Model file for the job. Use its own axes, mm. A direction names the side the tool comes from. Round coordinates to 2 decimals unless told otherwise and drop trailing zeros. Write each loop counter-clockwise with the first axis right and the second up, starting at its lowest first coordinate (ties: lowest second). Pieces come first, ordered by that corner, then holes. Notation, with made-up numbers: (77.5, 80) - (93.5, 80) arc R29 cw to (93.5, 108) - close; hole circle Ø9 at (-37.75, 24.5). An arc over 180 degrees is marked (long way). One line per item, written item: value.
from build123d import *

# Parameters (mm, degrees)
F1_DEPTH = 7.5
F2_W     = 18
F2_H     = 4
F2_W_2   = 8
F3_DEPTH = 7.5
F4_DEPTH = 5
F5_DEPTH = 25
F6_DEPTH = 3.5
F7_DEPTH = 25
F8_R     = 7
F9_R     = 1.99999


# Not quite as in the source:
# - a fillet or chamfer is up to 0.001 mm smaller than in the source, because OpenCascade refuses the exact size


with BuildPart() as f1:
    # F0 (on Top) → F1 (new body, symmetric)
    with BuildSketch(Plane.XY):
        Polygon((29.4704200836, 10.5355388032), (29.4704200836, 14.5355388032), (-5.5295799164, 14.5355388032), (-5.5295799164, -27.9644611968), (29.4704200836, -27.9644611968), (29.4704200836, -23.9644611968), (27.4704200836, -23.9644611968), (-1.5295799164, -23.9644611968), (-1.5295799164, 10.5355388032), (27.4704200836, 10.5355388032), align=None)
    extrude(amount=F1_DEPTH, both=True)

    # F2 (on Top) → F3 (join, symmetric)
    with BuildSketch(Plane.XY):
        Polygon((-30.5295799164, 18.5355388032), (-30.5295799164, 64.5355388032), (-18.5295799164, 64.5355388032), (-18.5295799164, 68.5355388032), (-34.5295799164, 68.5355388032), (-34.5295799164, 14.5355388032), (-23.5295799164, 14.5355388032), (-23.5295799164, 18.5355388032), align=None)
        Polygon((-10.5295799164, 68.5355388032), (-10.5295799164, 64.5355388032), (15.4704200836, 64.5355388032), (15.4704200836, 18.5355388032), (-5.5295799164, 18.5355388032), (-5.5295799164, 14.5355388032), (19.4704200836, 14.5355388032), (19.4704200836, 68.5355388032), align=None)
        with Locations((-14.5295799164, 16.5355388032)):
            Rectangle(F2_W, F2_H)
        with Locations((-14.5295799164, 66.5355388032)):
            Rectangle(F2_W_2, F2_H)
    extrude(amount=F3_DEPTH, both=True)

    # F2 (on Top) → F4 (cut, symmetric)
    with BuildSketch(Plane.XY):
        with Locations((-14.5295799164, 16.5355388032)):
            Rectangle(F2_W, F2_H)
    extrude(amount=F4_DEPTH, both=True, mode=Mode.SUBTRACT)

    # F2 (on Top) → F5 (cut)
    with BuildSketch(Plane.XY):
        with Locations((-14.5295799164, 16.5355388032)):
            Rectangle(F2_W, F2_H)
    extrude(amount=-F5_DEPTH, mode=Mode.SUBTRACT)

    # F2 (on Top) → F6 (cut, symmetric)
    with BuildSketch(Plane.XY):
        with Locations((-14.5295799164, 66.5355388032)):
            Rectangle(F2_W_2, F2_H)
    extrude(amount=F6_DEPTH, both=True, mode=Mode.SUBTRACT)

    # F2 (on Top) → F7 (cut)
    with BuildSketch(Plane.XY):
        with Locations((-14.5295799164, 66.5355388032)):
            Rectangle(F2_W_2, F2_H)
    extrude(amount=-F7_DEPTH, mode=Mode.SUBTRACT)

    # F8
    f8_edges = [f1.edges().sort_by_distance(p)[0] for p in [
        (-30.52958, 64.535539, 0),
        (15.47042, 64.535539, 0),
        (-30.52958, 18.535539, 0),
        (15.47042, 18.535539, 0),
    ]]
    fillet(f8_edges, radius=F8_R)

    # F9 (radius 2 in the source; OpenCascade refuses exactly that, so slightly less here)
    f9_edges = [f1.edges().sort_by_distance(p)[0] for p in [
        (19.47042, 41.535539, 7.5),
        (19.47042, 41.535539, -7.5),
        (24.47042, 14.535539, 7.5),
        (24.47042, 14.535539, -7.5),
        (19.47042, 68.535539, 0),
        (4.47042, 68.535539, -7.5),
        (-7.52958, 68.535539, 7.5),
        (-14.52958, 68.535539, 3.5),
        (-18.52958, 68.535539, -2),
        (-10.52958, 68.535539, -2),
        (-10.52958, 64.535539, -2),
        (-18.52958, 64.535539, -2),
        (-34.52958, 68.535539, 0),
        (-26.52958, 68.535539, -7.5),
        (-30.52958, 41.535539, -7.5),
        (15.47042, 41.535539, -7.5),
        (-34.52958, 41.535539, -7.5),
        (-29.02958, 14.535539, -7.5),
        (-34.52958, 41.535539, 7.5),
        (-20.02958, 14.535539, 7.5),
        (-30.52958, 41.535539, 7.5),
        (-23.52958, 14.535539, -1.25),
        (-5.52958, 18.535539, -1.25),
        (-5.52958, -4.714461, -7.5),
        (-5.52958, -6.714461, 7.5),
        (29.47042, -27.964461, 0),
        (-5.52958, -27.964461, 0),
        (-34.52958, 14.535539, 0),
        (29.47042, 14.535539, 0),
        (-21.02958, 64.535539, -7.5),
        (-28.479327, 62.485286, -7.5),
        (-28.479327, 20.585791, -7.5),
        (-28.479327, 20.585791, 7.5),
        (-7.52958, 64.535539, 7.5),
        (-1.02958, 64.535539, -7.5),
        (-28.479327, 62.485286, 7.5),
        (-7.52958, 18.535539, 7.5),
        (13.420168, 20.585791, 7.5),
        (13.420168, 62.485286, 7.5),
        (15.47042, 41.535539, 7.5),
        (1.47042, 18.535539, -7.5),
        (13.420168, 62.485286, -7.5),
        (13.420168, 20.585791, -7.5),
    ]]
    fillet(f9_edges, radius=F9_R)


solid = f1.part
1. Wall check: probe 1 along Y at (x, z) = (7.5, 2.5); probe 2 along X at (y, z) = (29, 5); probe 3 along Y at (x, z) = (21.5, 0). Give the ranges that are in metal, low to high. Write a range as [from, to].
Report:
probe 1: [-27.96, -23.96], [10.54, 18.54], [64.54, 68.54]
probe 2: [-34.53, -30.53], [15.47, 19.47]
probe 3: [-27.96, -23.96], [10.54, 14.54]
2. Drop flat-ended pins along their axis: pin 1 (0.6 mm diameter, centred on y = 17, z = -0.5, fed in from +X); pin 2 (9 mm diameter, centred on x = -22, z = -2, fed in from -Y); pin 3 (3.5 mm diameter, centred on y = -11, z = -1, fed in from -X). Give the stop position or say it passes through.
Report:
pin 1: x = 19.47
pin 2: y = 14.54
pin 3: x = -5.53
3. Tool access for faces 5 (the face through (23.386, 13.934, 6.93)), 6 (the face through (-4, 64.536, 0)), 7 (the face through (14, 10.536, 0)), 8 (the face through (-17.83, 15.14, 6.93)), 9 (the face through (16.04, 41.31, 6.9)): list every direction of +Z, -Z, +X, -X, +Y, -Y with a clear straight run to the whole face (end or side of a thin tool).
Report:
face 5: +Z, +X, +Y
face 6: +Z, -Z
face 7: +Z, -Z, +X
face 8: +Z, -X, -Y
face 9: +Z
4. Band-saw the part on C-C on y = -15.5. Write the cut outline in (x, z), plus the area to 3 significant figures.
Report:
outline: (-5.53, -5.5) arc R2 ccw to (-3.53, -7.5) - (-1.53, -7.5) - (-1.53, 7.5) - (-3.53, 7.5) arc R2 ccw to (-5.53, 5.5) - close
area: 58.3 mm²
5. Band-saw the part on B-B on x = 25. Write the cut outline in (y, z).
Report:
outline: (-27.96, -7.5) - (-23.96, -7.5) - (-23.96, 7.5) - (-27.96, 7.5) - close; (10.54, -7.5) - (12.54, -7.5) arc R2 ccw to (14.54, -5.5) - (14.54, 5.5) arc R2 ccw to (12.54, 7.5) - (10.54, 7.5) - close
6. Mould opens along Y. For faces 1 (the face through (23.386, 13.965, -6.899)), 2 (the face through (16.04, 41.31, -6.9)), 3 (the face through (8, 13, 7.5)), 4 (the face through (-21.55, 65.11, -6.9)) say: released by +Y, released by -Y, zero draft, split by the parting line, or undercut.
Report:
face 1: released by +Y
face 2: undercut
face 3: zero draft
face 4: released by -Y
